The listing builds one solid part. Answer for the finished solid, in the listing's coordinates (mm). Face numbers are marked on the shaded views. A direction names the side the tool comes from. Coordinates: 2 decimals unless noted, no trailing zeros. Order: outer loops, then holes, each group sorted by start corner. A loop starts at its lowest first (then second) coordinate and runs counter-clockwise, first axis right, second up. Notation, with made-up numbers: (-23, -22.75) -> (-15, -22.75) arc R15 cw to (-15, -10.75) -> close; hole circle Ø10 at (30, -34.5). An arc over 180 degrees is marked (long way). Answer in a Markdown table with one row per item. Add a question column.
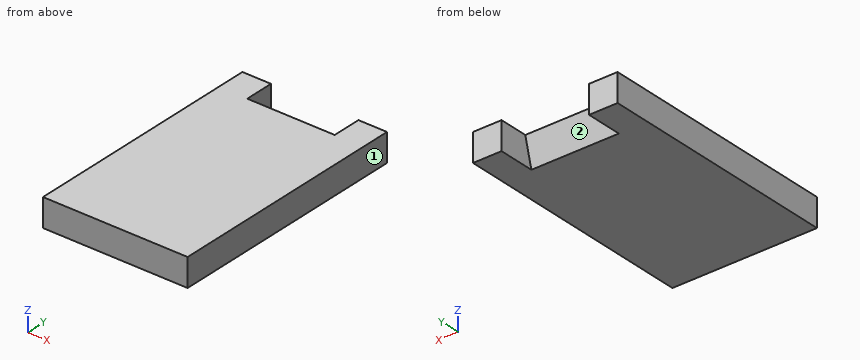
```python
from build123d import *

# Parameters (mm, degrees)
EXTRUDE_1_DEPTH = 9.6
DRAFT_5_ANGLE   = -15


with BuildPart() as part:
    # 草图1 → 凸台-拉伸1 (new body)
    with BuildSketch(Plane.XY):
        Polygon((9.8, 0), (0, 0), (0, -84.11), (49.6, -84.11), (49.6, 0), (39.8, 0), (39.8, -10), (9.8, -10), align=None)
    extrude(amount=EXTRUDE_1_DEPTH)

    # 拔模5
    draft_5_faces = [part.faces().sort_by_distance(p)[0] for p in [
        (24.8, -10, 4.8),
    ]]
    draft(draft_5_faces, Plane.XY.offset(9.6), DRAFT_5_ANGLE)


solid = part.part
```
Q1. Straight lines are drawn through the part: line 1 (X direction, y = -10.5, z = 2.5); line 2 (Y direction, x = 22, z = 5.75); line 3 (Y direction, x = 10, z = 3.75). For each, find the intervals that lie inside material, in ascending order.
Q2. A cutting plane is placed at A-A (y = -6). Determine the outline of the cut face in (x, z).
Q3. Given pin 1 (1.5 mm diameter, centred on x = 14, z = 7.5, fed in from +Y); pin 2 (4 mm diameter, centred on x = 37, z = 4.5, fed in from +Y), each flat-ended and moving along its own axis, determine where each tip first touches the part or whether it passes through.
Q4. A cutting plane is placed at C-C (x = 22.5). Determine the outline of the cut face in (y, z).
Q5. For the marked faces 1 and 2, determine the directions among +Z, -Z, +X, -X, +Y, -Y from which every point of the face is accessible in a straight line to the end or side of a thin tool.
Q6. A cutting plane is placed at B-B (z = 1.5). Determine the outline of the cut face in (x, y), then the cut area to 3 significant figures.
Returned:
| question | item | result |
|---|---|---|
| 1 | line 1 | x = 0 to 9.8, 39.8 to 49.6 |
| 1 | line 2 | y = -84.11 to -11.03 |
| 1 | line 3 | y = -84.11 to -11.57 |
| 2 | outline | (0, 0) -> (9.8, 0) -> (9.8, 9.6) -> (0, 9.6) -> close; (39.8, 0) -> (49.6, 0) -> (49.6, 9.6) -> (39.8, 9.6) -> close |
| 3 | pin 1 | stops at y = -10.36 |
| 3 | pin 2 | stops at y = -10.83 |
| 4 | outline | (-84.11, 0) -> (-12.57, 0) -> (-10, 9.6) -> (-84.11, 9.6) -> close |
| 5 | face 1 | +Z, -Z, +X, +Y, -Y |
| 5 | face 2 | -Z, +Y |
| 6 | outline | (0, -84.11) -> (49.6, -84.11) -> (49.6, 0) -> (39.8, 0) -> (39.8, -12.17) -> (9.8, -12.17) -> (9.8, 0) -> (0, 0) -> close |
| 6 | area | 3,810 mm² |
